Can you work these out from the model? Positions are in its coordinate system, mm. A direction names the side the tool comes from. Coordinates: 2 decimals unless noted, no trailing zeros. Use a Markdown table: item, result. Add a question column.
(1) For pin 1 Ø1 at (x, z) = (-23, 37) entering from +Y; pin 2 Ø2.5 at (x, z) = (-29.5, 72.39) entering from +Y; pin 3 Ø0.8 at (x, y) = (-2.5, -1.5) entering from -Z; pin 4 Ø0.8 at (x, y) = (-1, 0.5) entering from +Z (3 decimals), each with a flat end and sliding along its axis, tell me the tip position at first contact or that it passes through.
(2) I want a section at C-C (z = 72.39). State how many separate pieces and enclosed holes the cut face has, and give its area (3 significant figures).
(3) We'd pull the mould along Z, two halves only. Please class faces 1 (the cylindrical face through (29.08, -0.45, 0.59)), 2 (the flat face through (0, -2, 76.2)), 3 (the flat face through (-12.066, -2, 72)), 4 (the flat face through (0, -0.374, 75)): pulls with the +Z half, pulls with the -Z half, needs draft (parallel to the pull), parting line crosses it, or undercut.
(4) If I drill on L1, parallel to X at y = -0.8, z = 72.39; L2, parallel to X at y = -0.2, z = 61; L3, parallel to X at y = -0.8, z = 30, over which ranges is the centre line in solid material (lowest first)? Write a range as [from, to].
(5) On a 3-axis mill with a long thin cutter (end or side, diameter ignored), from which of +Z, -Z, +X, -X, +Y, -Y can I reach the whole of each face in a straight line? I mean faces 5 (the flat face through (-19.05, -2, 38)), 6 (the flat face through (-21, -3.175, 39)), 7 (the flat face through (-24, -0.374, 35)). Say none if no direction works.
Autodesk Inventor part; units mm, degrees
ref_plane "YZ Plane" through (0, 0, 0) normal (1, 0, 0) x (0, 1, 0)
ref_plane "XZ Plane" through (0, 0, 0) normal (0, 1, 0) x (-1, 0, 0)
ref_plane "XY Plane" through (0, 0, 0) normal (0, 0, 1) x (1, 0, 0)
sketch "Sketch1" plane through (0, 0, 0) normal (0, 0, 1) x (1, 0, 0)
  line L0 (-31.75, 5.08) -> (31.75, 5.08)
  line L1 (31.75, 5.08) -> (31.75, -5.08)
  line L2 (31.75, -5.08) -> (-31.75, -5.08)
  line L3 (-31.75, -5.08) -> (-31.75, 5.08)
  point P0 (0, 0)
  dimension "d0" = 63.5
  dimension "d3" = 31.75
  dimension "d4" = 10.16
  dimension "d17" = 5.08
extrude "Extrusion1" add sketch "Sketch1" along normal blind 76.2
sketch "Sketch3" plane through (0, 0, 76.2) normal (0, 0, 1) x (1, 0, 0)
  line L0 (-27.75, 0.3875) -> (27.75, 0.3875)
  line L1 (27.75, 0.3875) -> (27.75, -0.3745)
  line L2 (27.75, -0.3745) -> (-27.75, -0.3745)
  line L3 (-27.75, -0.3745) -> (-27.75, 0.3875)
  line L4 (-31.75, 5.08) -> (-31.75, -5.08)
  point P0 (0, 0)
  point P1 (-27.75, 0.0065)
  dimension "d6" = 0.762
  dimension "d7" = 55.5
  dimension "d8" = 4
extrude "Extrusion2" cut sketch "Sketch3" against normal blind 85.1
sketch "Sketch8" plane through (0, 0, 76.2) normal (0, 0, 1) x (1, 0, 0)
  line L0 (27.75, 0.3875) -> (27.75, -0.3745)
  line L1 (27.75, -0.3745) -> (-27.75, -0.3745)
  line L2 (-27.75, -0.3745) -> (-27.75, 0.3875)
  line L3 (-27.75, 0.3875) -> (27.75, 0.3875)
  line L4 (-31.75, -5.08) -> (31.75, -5.08)
  line L5 (31.75, -5.08) -> (31.75, 5.08)
  line L6 (31.75, 5.08) -> (-31.75, 5.08)
  line L7 (-31.75, 5.08) -> (-31.75, -5.08)
  line L8 (-31.75, 5.08) -> (31.75, 5.08)
  line L9 (31.75, 5.08) -> (31.75, 0.3875)
  line L10 (31.75, 0.3875) -> (-31.75, 0.3875)
  line L11 (-31.75, 0.3875) -> (-31.75, 5.08)
  point P0 (0, 0)
  point P1 (-31.75, 0.3875)
  dimension "d30" = 0
extrude "Extrusion6" cut sketch "Sketch8" against normal blind 76.2 contours L3 L10 L7 L6 L5
sketch "Sketch9" plane through (0, 0, 76.2) normal (0, 0, 1) x (1, 0, 0)
  line L0 (-31.75, 0.3875) -> (-31.75, -5.08)
  line L1 (31.75, -5.08) -> (31.75, 0.3875)
  line L2 (-31.75, -5.08) -> (31.75, -5.08)
  line L3 (31.75, -5.08) -> (31.75, -3.175)
  line L4 (31.75, -3.175) -> (-31.75, -3.175)
  line L5 (-31.75, -3.175) -> (-31.75, -5.08)
  point P0 (0, 0)
  dimension "d33" = 1.905
extrude "Extrusion7" cut sketch "Sketch9" against normal blind 76.2
sketch "Sketch10" plane through (-27.75, -0.3745, 76.2) normal (0, 1, 0) x (1, 0, 0)
  line L0 (59.5, 76.2) -> (-4, 76.2)
  line L1 (-4, 76.2) -> (59.5, 76.2)
  line L2 (59.5, 76.2) -> (59.5, 0)
  line L3 (59.5, 0) -> (-4, 0)
  line L4 (-4, 0) -> (-4, 76.2)
  line L5 (8.7, 12.7) -> (46.8, 12.7)
  line L6 (46.8, 12.7) -> (46.8, 63.5)
  line L7 (46.8, 63.5) -> (8.7, 63.5)
  line L8 (8.7, 63.5) -> (8.7, 12.7)
  dimension "d46" = 12.7
extrude "Extrusion8" cut sketch "Sketch10" against normal blind 25.4 contours L8 L7 L6 L5
fillet "Fillet3" radius 3.175 3 edges at (0, -0.3745, 0) (-27.75, 0.0065, 0) (27.75, 0.0065, 0)
sketch "Sketch11" plane through (-27.75, -0.3745, 76.2) normal (0, 1, 0) x (1, 0, 0)
  line L0 (15.6845, 1.905) -> (39.8145, 1.905)
  line L1 (39.8145, 1.905) -> (39.8145, 5.715)
  line L2 (39.8145, 5.715) -> (15.6845, 5.715)
  line L3 (15.6845, 5.715) -> (15.6845, 1.905)
  line L4 (55.5, 0) -> (0, 0)
  line L5 (0, 0) -> (0, 73.025)
  line L6 (-4, 0) -> (-4, 76.2)
  point P0 (27.75, 76.2)
  dimension "d47" = 1.905
  dimension "d48" = 3.81
  dimension "d51" = 24.13
  dimension "d52" = 15.6845
  dimension "d67" = 19.6845
extrude "Extrusion9" cut sketch "Sketch11" against normal blind 25.4
sketch "Sketch13" plane through (-31.75, -3.175, 76.2) normal (0, -1, 0) x (1, 0, 0)
  circle A0 centre (61.25, -3.81) radius 1.05
  line L0 (63.5, 0) -> (59, 0)
  circle A1 centre (2.25, -3.81) radius 1.05
  line L1 (4.5, 0) -> (0, 0)
  circle A2 centre (61.25, -72.39) radius 1.05
  line L2 (59, -76.2) -> (63.5, -76.2)
  line L3 (59, 0) -> (59, -76.2)
  circle A3 centre (2.25, -72.39) radius 1.05
  line L4 (0, 0) -> (0, -76.2)
  line L5 (0, -76.2) -> (4.5, -76.2)
  line L6 (50.8, -12.7) -> (50.8, -63.5)
  line L7 (50.8, -63.5) -> (12.7, -63.5)
  line L8 (12.7, -63.5) -> (12.7, -12.7)
  line L9 (12.7, -12.7) -> (50.8, -12.7)
  line L10 (63.5, 0) -> (0, 0)
  line L11 (0, 0) -> (0, -76.2)
  line L12 (63.5, -76.2) -> (0, -76.2)
  line L13 (63.5, 0) -> (63.5, -76.2)
  point P0 (31.75, -76.2)
  point P1 (31.75, -76.2)
  dimension "d53" = 2.1
  dimension "d54" = 3.81
  dimension "d55" = 2.25
  dimension "d56" = 2.25
  dimension "d57" = 2.1
  dimension "d58" = 3.81
  dimension "d59" = 2.1
  dimension "d60" = 2.1
  dimension "d61" = 3.81
  dimension "d62" = 3.81
  dimension "d63" = 2.25
  dimension "d64" = 2.25
extrude "Extrusion10" cut sketch "Sketch13" against normal blind 25.4 contours A0 | A1 | A2 | A3
sketch "Sketch14" plane through (-31.75, 0.3875, 76.2) normal (0, 1, 0) x (1, 0, 0)
  circle A0 centre (2.25, 3.81) radius 1.05
  circle A1 centre (2.25, 72.39) radius 1.05
  arc A2 (4, 73.025) -> (0.825, 76.2) centre (0.825, 73.025) ccw
  line L0 (0, 76.2) -> (0.825, 76.2)
  line L1 (0, 0) -> (0, 76.2)
  line L2 (4, 0) -> (0, 0)
  line L3 (4, 0) -> (4, 73.025)
  circle A3 centre (61.25, 3.81) radius 1.05
  circle A4 centre (61.25, 72.39) radius 1.05
  arc A5 (62.675, 76.2) -> (59.5, 73.025) centre (62.675, 73.025) ccw
  line L4 (59.5, 0) -> (59.5, 73.025)
  line L5 (63.5, 0) -> (59.5, 0)
  line L6 (63.5, 76.2) -> (63.5, 0)
  line L7 (62.675, 76.2) -> (63.5, 76.2)
  point P0 (31.75, 76.2)
extrude "Extrusion11" add sketch "Sketch14" along normal blind 0.5
sketch "Sketch15" plane through (-27.75, -0.3745, 76.2) normal (0, 1, 0) x (1, 0, 0)
  line L0 (0, 0) -> (0, 73.025)
  line L1 (0, 6.715) -> (55.7227, 6.715)
  line L2 (55.7227, 6.715) -> (55.7227, 9.255)
  line L3 (55.7227, 9.255) -> (0, 9.255)
  line L4 (0, 9.255) -> (0, 6.715)
  line L5 (15.6845, 5.715) -> (39.8145, 5.715)
  point P0 (27.75, 76.2)
  point P1 (0, 9.255)
  dimension "d72" = 2.54
  dimension "d77" = 1
extrude "Extrusion12" add sketch "Sketch15" along normal blind 1.3
sketch "Sketch16" plane through (0, 0, 76.2) normal (0, 0, 1) x (1, 0, 0)
  line L0 (31.75, -3.175) -> (31.75, 0.8875)
  line L1 (-36.1102, 11.8694) -> (32.0392, 11.8694)
  line L2 (32.0392, 11.8694) -> (32.0392, 0.6335)
  line L3 (32.0392, 0.6335) -> (-36.1102, 0.6335)
  line L4 (-36.1102, 0.6335) -> (-36.1102, 11.8694)
  line L5 (-31.75, 0.8875) -> (-27.75, 0.8875)
  point P0 (0, 0)
  dimension "d79" = 0.254
extrude "Extrusion13" cut sketch "Sketch16" against normal blind 254
sketch "Sketch18" plane through (0, 0, 0) normal (0, 0, -1) x (-1, 0, 0)
  line L0 (27.7501, -0.3745) -> (-27.7501, -0.3745)
  line L1 (27.75, 0.6335) -> (-27.75, 0.6335)
  point P0 (0, 0)
  dimension "d78" = 1.008
properties part number "Scanner_Test_Bot"
Answers follow:
| question | item | result |
|---|---|---|
| 1 | pin 1 | stops at y = -0.37 |
| 1 | pin 2 | stops at y = 0.63 |
| 1 | pin 3 | stops at z = 0.44 |
| 1 | pin 4 | stops at z = 69.485 |
| 2 | separate pieces | 4 |
| 2 | enclosed holes | 0 |
| 2 | area | 102 mm² |
| 3 | face 1 | pulls with the -Z half |
| 3 | face 2 | pulls with the +Z half |
| 3 | face 3 | undercut |
| 3 | face 4 | needs draft |
| 4 | L1 | x = [-31.75, -30.55], [-28.45, -12.07], [12.06, 28.45], [30.55, 31.75] |
| 4 | L2 | x = [-31.75, -27.75], [27.75, 31.75] |
| 4 | L3 | x = [-31.75, -19.05], [19.05, 31.75] |
| 5 | face 5 | +Y, -Y |
| 5 | face 6 | +Z, -Z, +X, -X, -Y |
| 5 | face 7 | -Z, +Y |
